from build123d import *

# Parameters (mm, degrees)
BOSS_EXTRUDE1_DEPTH = 8
SKETCH5_W           = 160
SKETCH5_H           = 8
BOSS_EXTRUDE4_DEPTH = 10
SKETCH6_W           = 20
SKETCH6_H           = 8
BOSS_EXTRUDE5_DEPTH = 8
SKETCH7_R           = 4
CUT_EXTRUDE2_DEPTH  = 8


with BuildPart() as part:
    # Sketch1 → Boss-Extrude1 (new body)
    with BuildSketch(Plane.XY):
        with BuildLine():
            Line((-80, 0), (80, 0))
            ThreePointArc((80, 0), (0, 80), (-80, 0))
        make_face()
    extrude(amount=BOSS_EXTRUDE1_DEPTH)

    # Sketch5 → Boss-Extrude4 (add)
    with BuildSketch(Plane.XZ):
        with Locations((0, 4)):
            Rectangle(SKETCH5_W, SKETCH5_H)
    extrude(amount=BOSS_EXTRUDE4_DEPTH)

    # Sketch6 → Boss-Extrude5 (add)
    with BuildSketch(Plane.XZ.offset(10)):
        with Locations((-70, 4)):
            Rectangle(SKETCH6_W, SKETCH6_H)
    boss_extrude5 = extrude(amount=BOSS_EXTRUDE5_DEPTH)

    # Mirror2: Boss-Extrude5 across plane
    add(boss_extrude5.mirror(Plane(origin=(0, 0, 0), x_dir=(0, 0, 1), z_dir=(1, 0, 0))))

    # Sketch7 → Cut-Extrude2 (cut)
    with BuildSketch(Plane.XY.offset(8)):
        Circle(SKETCH7_R)
    extrude(amount=-CUT_EXTRUDE2_DEPTH, mode=Mode.SUBTRACT)


solid = part.part
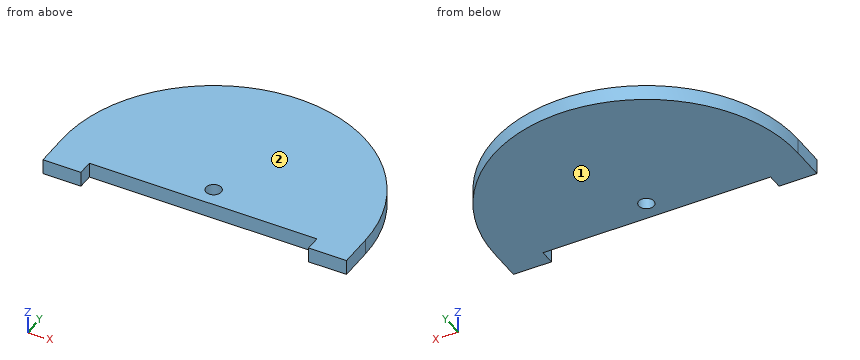
Here's how the part is built. I have some questions about the finished solid (model axes, mm). Face numbers are marked on the shaded views. Round coordinates to 2 decimals unless told otherwise and drop trailing zeros. Write each loop counter-clockwise with the first axis right and the second up, starting at its lowest first coordinate (ties: lowest second). Pieces come first, ordered by that corner, then holes.
1. Will these pins go through, and if not, where does the flat tip stop? pin 1 Ø1.5 at (x, z) = (59.5, 5.5) entering from +Y; pin 2 Ø1.5 at (x, z) = (-26, 6) entering from -Y; pin 3 Ø3 at (y, z) = (49, 6) entering from -X.
2. Suppose I cut it at B-B (z = 2.25). List the corners of the cut face in (x, y) for me.
3. Suppose I cut it at C-C (y = 64). List the corners of the cut face in (x, z) for me, and give its area (3 significant figures).
4. Suppose I cut it at A-A (x = 0). List the corners of the cut face in (y, z) for me, and give its area (3 significant figures).
5. If we mould it in two halves opening along Z, with no side actions, what happens to the marked faces 1 and 2? For each: released by +Z, released by -Z, zero draft, split by the parting line, or undercut.
6. I need wall thicknesses on L1, parallel to Y at x = 0, z = 3.25; L2, parallel to X at y = 1, z = 6.5; L3, parallel to Y at x = 51.5, z = 6. Which ranges of each line are inside material? Lowest first, please.
7. Suppose I cut it at D-D (x = -21). List the corners of the cut face in (y, z) for me, and give its area (3 significant figures).
Answer sheet:
1. pin 1: stops at y = 54.3
1. pin 2: stops at y = -10
1. pin 3: stops at x = -64.37
2. outline: (-80, -18) - (-60, -18) - (-60, -10) - (60, -10) - (60, -18) - (80, -18) - (80, 0) arc R80 ccw to (-80, 0) - close; hole circle Ø8 at (0, 0)
3. outline: (-48, 0) - (48, 0) - (48, 8) - (-48, 8) - close
3. area: 768 mm2
4. outline: (-10, 0) - (-4, 0) - (-4, 8) - (-10, 8) - close; (4, 0) - (80, 0) - (80, 8) - (4, 8) - close
4. area: 656 mm2
5. face 1: released by -Z
5. face 2: released by +Z
6. L1: y = -10 to -4, 4 to 80
6. L2: x = -79.99 to -3.87, 3.87 to 79.99
6. L3: y = -10 to 61.22
7. outline: (-10, 0) - (77.19, 0) - (77.19, 8) - (-10, 8) - close
7. area: 698 mm2
